CAD build for the part. Positions are in the model's coordinates, mm. Face numbers are marked on the shaded views. A direction names the side the tool comes from. Coordinates: 2 decimals unless noted, no trailing zeros. Write each loop counter-clockwise with the first axis right and the second up, starting at its lowest first coordinate (ties: lowest second). Pieces come first, ordered by that corner, then holes. Notation, with made-up numbers: (37.5, -8) -> (56.5, -8) arc R12 cw to (56.5, 9) -> close; hole circle Ø6 at (23.5, 68). An arc over 180 degrees is marked (long way). Answer as CSV lines item,"result".
Autodesk Inventor part; units mm, degrees
ref_plane "YZ Plane" through (0, 0, 0) normal (1, 0, 0) x (0, 1, 0)
ref_plane "XZ Plane" through (0, 0, 0) normal (0, 1, 0) x (-1, 0, 0)
ref_plane "XY Plane" through (0, 0, 0) normal (0, 0, 1) x (1, 0, 0)
sketch "Sketch1" plane through (0, 0, 0) normal (0, 1, 0) x (-1, 0, 0)
  line L0 (46.8376, 46.8376) -> (-46.8376, 46.8376)
  line L1 (-46.8376, 46.8376) -> (-46.8376, -46.8376)
  line L2 (-46.8376, -46.8376) -> (46.8376, -46.8376)
  line L3 (46.8376, -46.8376) -> (46.8376, 46.8376)
  line L4 (6.0071, 6.0071) -> (-6.0071, 6.0071) construction
  line L5 (-6.0071, 6.0071) -> (-6.0071, -6.0071) construction
  line L6 (-6.0071, -6.0071) -> (6.0071, -6.0071) construction
  line L7 (6.0071, -6.0071) -> (6.0071, 6.0071) construction
  circle A0 centre (-40.0304, -40.0304) radius 2.159
  circle A1 centre (40.0304, -40.0304) radius 2.159
  circle A2 centre (40.0304, 40.0304) radius 2.159
  circle A3 centre (-40.0304, 40.0304) radius 2.159
  circle A4 centre (0, 0) radius 2.159
  point P0 (46.8376, 0)
  point P1 (0, -46.8376)
  point P2 (6.0071, 0)
  point P3 (0, -6.0071)
  dimension "d0" = 93.6752
  dimension "d1" = 12.0142
  dimension "d24" = 6.8072
  dimension "d25" = 6.8072
  dimension "d26" = 4.318
  dimension "d29" = 360
  dimension "d53" = 4.318
extrude "Extrusion1" add sketch "Sketch1" along normal blind 0.508
sketch "Sketch3" plane through (0, 0.508, 0) normal (0, 1, 0) x (1, 0, 0)
  line L0 (-6.0071, 6.0071) -> (6.0071, 6.0071) construction
  line L1 (6.0071, 6.0071) -> (6.0071, -6.0071) construction
  line L2 (6.0071, -6.0071) -> (-6.0071, -6.0071) construction
  line L3 (-6.0071, -6.0071) -> (-6.0071, 6.0071) construction
  line L4 (6.0071, 46.8376) -> (7.6073, 46.8376)
  line L5 (7.6073, 46.8376) -> (7.6073, 8.7376)
  line L6 (7.6073, 8.7376) -> (6.0071, 8.7376)
  line L7 (6.0071, 8.7376) -> (6.0071, 46.8376)
  line L8 (46.8376, 46.8376) -> (-46.8376, 46.8376)
  line L9 (-46.8376, 7.6073) -> (-8.7376, 7.6073)
  line L10 (-8.7376, 6.0071) -> (-46.8376, 6.0071)
  line L11 (-8.7376, 7.6073) -> (-8.7376, 6.0071)
  line L12 (-46.8376, 6.0071) -> (-46.8376, 7.6073)
  line L13 (-7.6073, -46.8376) -> (-7.6073, -8.7376)
  line L14 (-6.0071, -8.7376) -> (-6.0071, -46.8376)
  line L15 (-7.6073, -8.7376) -> (-6.0071, -8.7376)
  line L16 (-6.0071, -46.8376) -> (-7.6073, -46.8376)
  line L17 (46.8376, -7.6073) -> (8.7376, -7.6073)
  line L18 (8.7376, -6.0071) -> (46.8376, -6.0071)
  line L19 (8.7376, -7.6073) -> (8.7376, -6.0071)
  line L20 (46.8376, -6.0071) -> (46.8376, -7.6073)
  line L21 (-6.0071, 17.533) -> (-4.8756, 18.6645)
  line L22 (-4.8756, 18.6645) -> (4.1047, 9.6843)
  line L23 (4.1047, 9.6843) -> (2.9732, 8.5528)
  line L24 (2.9732, 8.5528) -> (-6.0071, 17.533)
  line L25 (0, 0) -> (-6.0071, 0) construction
  line L26 (-18.6645, -4.8756) -> (-9.6843, 4.1047)
  line L27 (-17.533, -6.0071) -> (-18.6645, -4.8756)
  line L28 (-8.5528, 2.9732) -> (-17.533, -6.0071)
  line L29 (-9.6843, 4.1047) -> (-8.5528, 2.9732)
  line L30 (4.8756, -18.6645) -> (-4.1047, -9.6843)
  line L31 (6.0071, -17.533) -> (4.8756, -18.6645)
  line L32 (-2.9732, -8.5528) -> (6.0071, -17.533)
  line L33 (-4.1047, -9.6843) -> (-2.9732, -8.5528)
  line L34 (18.6645, 4.8756) -> (9.6843, -4.1047)
  line L35 (17.533, 6.0071) -> (18.6645, 4.8756)
  line L36 (8.5528, -2.9732) -> (17.533, 6.0071)
  line L37 (9.6843, -4.1047) -> (8.5528, -2.9732)
  line L38 (37.4904, -7.6073) -> (42.5704, -7.6073)
  line L39 (42.5704, -7.6073) -> (42.5704, -35.631)
  line L40 (37.4904, -35.631) -> (37.4904, -7.6073)
  line L41 (-6.0071, -37.4904) -> (35.631, -37.4904)
  line L42 (35.631, -42.5704) -> (-6.0071, -42.5704)
  line L43 (-6.0071, -42.5704) -> (-6.0071, -37.4904)
  line L44 (0.2495, 13.5394) -> (6.0071, 13.5394)
  line L45 (6.0071, 13.5394) -> (6.0071, 14.8094)
  line L46 (6.0071, 14.8094) -> (-1.0205, 14.8094)
  line L47 (-13.5394, 0.2495) -> (-13.5394, 6.0071)
  line L48 (-14.8094, 6.0071) -> (-14.8094, -1.0205)
  line L49 (-0.2495, -13.5394) -> (-6.0071, -13.5394)
  line L50 (-6.0071, -14.8094) -> (1.0205, -14.8094)
  line L51 (13.5394, -0.2495) -> (13.5394, -6.0071)
  line L52 (14.8094, -6.0071) -> (14.8094, 1.0205)
  circle A0 centre (-40.0304, 40.0304) radius 2.159
  circle A1 centre (40.0304, -40.0304) radius 2.159
  line L53 (37.4904, -7.6073) -> (42.5704, -7.6073)
  arc A2 (35.631, -42.5704) -> (42.5704, -35.631) centre (40.0304, -40.0304) ccw
  arc A3 (37.4904, -35.631) -> (35.631, -37.4904) centre (40.0304, -40.0304) ccw
  line L54 (-42.5704, 7.6073) -> (-42.5704, 35.631)
  arc A4 (-35.631, 42.5704) -> (-42.5704, 35.631) centre (-40.0304, 40.0304) ccw
  line L55 (6.0071, 37.4904) -> (-35.631, 37.4904)
  line L56 (-35.631, 42.5704) -> (6.0071, 42.5704)
  arc A5 (-37.4904, 35.631) -> (-35.631, 37.4904) centre (-40.0304, 40.0304) ccw
  line L57 (-37.4904, 35.631) -> (-37.4904, 7.6073)
  circle A6 centre (0, 0) radius 3.1458
  point P0 (0, 6.0071)
  point P1 (6.0071, 0)
  point P2 (-1.517, 13.0429)
  point P3 (-13.0429, -1.517)
  point P4 (1.517, -13.0429)
  point P5 (13.0429, 1.517)
  point P6 (-0.3855, 14.1744)
  point P7 (6.0071, 14.1744)
  point P8 (40.0304, -7.6073)
  point P9 (-6.0071, -40.0304)
  point P10 (14.8094, 1.0205)
  point P11 (-6.0071, -13.5394)
  point P12 (-6.0071, -42.5704)
  point P13 (-14.8094, -1.0205)
  point P14 (6.0071, 42.5704)
  dimension "d8" = 12.0142
  dimension "d9" = 1.6002
  dimension "d10" = 38.1
  dimension "d13" = 360
  dimension "d15" = 1.6002
  dimension "d16" = 12.7
  dimension "d17" = 45
  dimension "d19" = 7.0358
  dimension "d22" = 360
  dimension "d31" = 1.27
  dimension "d34" = 360
  dimension "d40" = 5.08
  dimension "d41" = 5.08
  dimension "d42" = 5.08
  dimension "d43" = 5.08
  dimension "d46" = 180
  dimension "d55" = 6.2916
extrude "Extrusion4" cut sketch "Sketch3" against normal blind 2.54 contours L4 L5 L6 L7 | L9 L11 L10 L12 | L13 L15 L14 L16 | L17 L19 L18 L20 keep common part
sketch "Sketch6" plane through (-7.6073, 0, 46.8376) normal (0, 0, 1) x (1, 0, 0)
  line L0 (0, 0.508) -> (1.6002, 0.508)
  line L1 (0.8001, 0.508) -> (0, 0.254)
  line L2 (0, 0.508) -> (0, 0)
  line L3 (0.8001, 0.508) -> (1.6002, 0.254)
  line L4 (1.6002, 0.508) -> (1.6002, 0)
  line L5 (15.2146, 0.508) -> (13.6144, 0.508)
  line L6 (14.4145, 0.508) -> (13.6144, 0.254)
  line L7 (13.6144, 0.508) -> (13.6144, 0)
  line L8 (14.4145, 0.508) -> (15.2146, 0.254)
  line L9 (15.2146, 0.508) -> (15.2146, 0)
  line L10 (0, 0.254) -> (0, 0.508)
  line L11 (1.6002, 0.508) -> (1.6002, 0.254)
  line L12 (13.6144, 0.254) -> (13.6144, 0.508)
  line L13 (15.2146, 0.508) -> (15.2146, 0.254)
  point P0 (7.6073, 0)
extrude "Extrusion5" cut sketch "Sketch6" against normal through all
sketch "Sketch7" plane through (-46.8376, 0, -7.6073) normal (-1, 0, 0) x (0, 0, 1)
  line L0 (0, 0.508) -> (1.6002, 0.508)
  line L1 (0.8001, 0.508) -> (0, 0.254)
  line L2 (0, 0.508) -> (0, 0)
  line L3 (0.8001, 0.508) -> (1.6002, 0.254)
  line L4 (1.6002, 0.508) -> (1.6002, 0)
  line L5 (1.6002, 0.254) -> (1.6002, 0.508)
  line L6 (1.6002, 0.508) -> (0, 0.508)
  line L7 (0, 0.508) -> (0, 0.254)
  line L8 (15.2146, 0.508) -> (13.6144, 0.508)
  line L9 (14.4145, 0.508) -> (13.6144, 0.254)
  line L10 (13.6144, 0.508) -> (13.6144, 0)
  line L11 (14.4145, 0.508) -> (15.2146, 0.254)
  line L12 (15.2146, 0.508) -> (15.2146, 0)
  line L13 (15.2146, 0.254) -> (15.2146, 0.508)
  line L14 (15.2146, 0.508) -> (13.6144, 0.508)
  line L15 (13.6144, 0.508) -> (13.6144, 0.254)
  point P0 (7.6073, 0)
extrude "Extrusion6" cut sketch "Sketch7" against normal through all
sketch "Sketch9" plane through (0, 0, 0) normal (0, -1, 0) x (1, 0, 0)
  line L0 (-8.89, 8.89) -> (8.89, 8.89)
  line L1 (8.89, 8.89) -> (8.89, -8.89)
  line L2 (8.89, -8.89) -> (-8.89, -8.89)
  line L3 (-8.89, -8.89) -> (-8.89, 8.89)
  circle A0 centre (0, 0) radius 2.159
  line L4 (46.8376, 6.0071) -> (8.7376, 6.0071)
  line L5 (17.1195, 6.0071) -> (8.89, 1.4168)
  line L6 (22.1995, 6.0071) -> (8.89, -1.4168)
  line L7 (17.1195, 6.0071) -> (22.1995, 6.0071)
  line L8 (8.89, 1.4168) -> (8.89, -1.4168)
  line L9 (-6.0071, 17.1195) -> (-1.4168, 8.89)
  line L10 (-6.0071, 22.1995) -> (1.4168, 8.89)
  line L11 (-6.0071, 17.1195) -> (-6.0071, 22.1995)
  line L12 (-17.1195, -6.0071) -> (-8.89, -1.4168)
  line L13 (-22.1995, -6.0071) -> (-8.89, 1.4168)
  line L14 (-17.1195, -6.0071) -> (-22.1995, -6.0071)
  line L15 (6.0071, -17.1195) -> (1.4168, -8.89)
  line L16 (6.0071, -22.1995) -> (-1.4168, -8.89)
  line L17 (6.0071, -17.1195) -> (6.0071, -22.1995)
  point P0 (0, 8.89)
  point P1 (8.89, 0)
  point P2 (8.89, 0)
  point P3 (-1.4168, -8.89)
  point P4 (1.4168, 8.89)
  dimension "d62" = 17.78
  dimension "d63" = 4.318
  dimension "d65" = 5.08
  dimension "d66" = 15.24
  dimension "d69" = 360
extrude "Extrusion7" add sketch "Sketch9" against normal blind 0.254 contours L0 L1 L2 L3 | L9 L11 L10 L0 | L3 L12 L14 L13 | L2 L15 L17 L16 | L5 L4 L6 L1
properties part number "FlasherGuide"
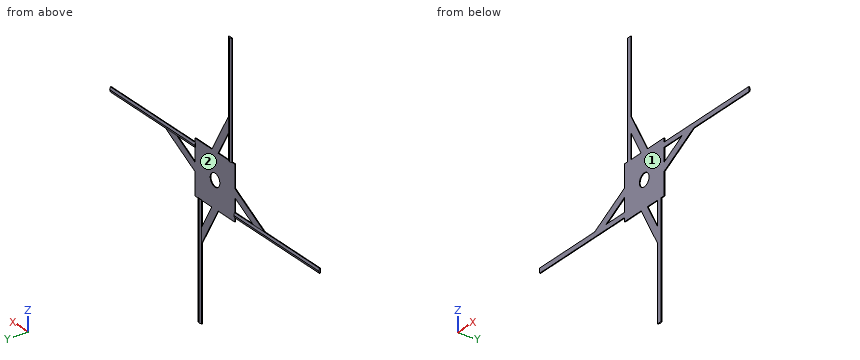
Item 1: Saw through at C-C on x = 33.5. Give the cut face in (y, z), and give its area (3 significant figures).
Answer below:
outline,"(0, 6.01) -> (0.25, 6.01) -> (0.51, 6.81) -> (0.25, 7.61) -> (0, 7.61) -> close"
area,"0.610 mm2"
Item 2: 3-axis set-ups, long thin cutter, end or side, ignore diameter. For the marked faces 1 and 2: which of +Z, -Z, +X, -X, +Y, -Y reach the whole face in a straight line?
Answer below:
face 1,"+Z, -Z, +X, -X, -Y"
face 2,"+Y"
Item 3: Saw through at D-D on y = 0.1. State how many separate pieces and enclosed holes the cut face has, and give its area (3 significant figures).
Answer below:
separate pieces,"1"
enclosed holes,"5"
area,"666 mm2"
Item 4: Wall check: line 1 (Z direction, x = 0, y = 0.1); line 2 (X direction, y = 0.2, z = -4); line 3 (X direction, y = 0.2, z = -36). Give the ranges that are in metal, low to high. Write a range as from..to.
Answer below:
line 1,"z = -11.43..-2.16, 2.16..11.43"
line 2,"x = -18.6..-13.52, -8.89..8.89"
line 3,"x = 6.01..7.61"
Item 5: Saw through at A-A on x = 0. Give the cut face in (y, z), and give its area (3 significant figures).
Answer below:
outline,"(0, -11.43) -> (0.25, -11.43) -> (0.25, -2.16) -> (0, -2.16) -> close; (0, 2.16) -> (0.25, 2.16) -> (0.25, 11.43) -> (0, 11.43) -> close"
area,"4.71 mm2"
Item 6: Saw through at B-B on z = 0. Give the cut face in (x, y).
Answer below:
outline,"(-11.43, 0) -> (-2.16, 0) -> (-2.16, 0.25) -> (-11.43, 0.25) -> close; (2.16, 0) -> (11.43, 0) -> (11.43, 0.25) -> (2.16, 0.25) -> close"
